```python
from build123d import *

# Parameters (mm, degrees)
BOSS_EXTRUDE1_DEPTH                             = 2
SKETCH2_R                                       = 4.4
CUT_EXTRUDE1_DEPTH                              = 34.661067402
CUT_EXTRUDE2_REACH                              = 35.661
SKETCH5_R                                       = 1.5
CSK_FOR_M2_FLAT_HEAD_MACHINE_SCREW1_D           = 2.4
CSK_FOR_M2_FLAT_HEAD_MACHINE_SCREW1_DEPTH       = 42.93
CSK_FOR_M2_FLAT_HEAD_MACHINE_SCREW1_CSINK_D     = 4.4
CSK_FOR_M2_FLAT_HEAD_MACHINE_SCREW1_CSINK_ANGLE = 90
CSK_FOR_M2_FLAT_HEAD_MACHINE_SCREW1_TIP         = 0.721032743
CSK_FOR_M2_FLAT_HEAD_MACHINE_SCREW2_D           = 2.4
CSK_FOR_M2_FLAT_HEAD_MACHINE_SCREW2_DEPTH       = 42.93
CSK_FOR_M2_FLAT_HEAD_MACHINE_SCREW2_CSINK_D     = 4.4
CSK_FOR_M2_FLAT_HEAD_MACHINE_SCREW2_CSINK_ANGLE = 90
CSK_FOR_M2_FLAT_HEAD_MACHINE_SCREW2_TIP         = 0.721032743


with BuildPart() as part:
    # Sketch1 → Boss-Extrude1 (new body)
    with BuildSketch(Plane(origin=(0, 0, 0), x_dir=(1, 0, 0), z_dir=(0, 1, 0))):
        Polygon((-11.293051345, 29.704532022), (12.706948655, 29.704532022), (15.706948655, 26.704532022), (15.706948655, 2.704532022), (12.706948655, -0.295467978), (-11.293051345, -0.295467978), (-14.293051345, 2.704532022), (-14.293051345, 26.704532022), align=None)
    extrude(amount=BOSS_EXTRUDE1_DEPTH)

    # Sketch2 → Cut-Extrude1 (cut, through all)
    with BuildSketch(Plane(origin=(0, 2, 0), x_dir=(1, 0, 0), z_dir=(0, 1, 0))):
        with Locations(Location((0, 14.704532022, 0), (0, 0, 270))):
            Circle(SKETCH2_R)
    extrude(amount=-CUT_EXTRUDE1_DEPTH, mode=Mode.SUBTRACT)

    # Sketch5 → Cut-Extrude2 (cut, up to next)
    with BuildSketch(Plane(origin=(0, 2, 0), x_dir=(1, 0, 0), z_dir=(0, 1, 0)), mode=Mode.PRIVATE) as cut_extrude2_sk1:
        with Locations(Location((-3.508440786, 20.204532022, 0), (0, 0, 270))):
            Circle(SKETCH5_R)
    cut_extrude2_tool1 = extrude(cut_extrude2_sk1.sketch, amount=-CUT_EXTRUDE2_REACH, mode=Mode.PRIVATE) & part.part
    # Sketch5 → Cut-Extrude2 (cut, up to next)
    with BuildSketch(Plane(origin=(0, 2, 0), x_dir=(1, 0, 0), z_dir=(0, 1, 0)), mode=Mode.PRIVATE) as cut_extrude2_sk2:
        with Locations(Location((3.491559214, 20.204532022, 0), (0, 0, 270))):
            Circle(SKETCH5_R)
    cut_extrude2_tool2 = extrude(cut_extrude2_sk2.sketch, amount=-CUT_EXTRUDE2_REACH, mode=Mode.PRIVATE) & part.part
    add(cut_extrude2_tool1.solids().sort_by_distance((-3.508441, 2, -20.204532))[0], mode=Mode.SUBTRACT)
    add(cut_extrude2_tool2.solids().sort_by_distance((3.491559, 2, -20.204532))[0], mode=Mode.SUBTRACT)

    # CSK for M2 Flat Head Machine Screw1
    with Locations(Plane(origin=(-3.508440786, 2, -20.204532022), x_dir=(0, 0, 1), z_dir=(0, 1, 0))):
        with Locations((0, 0), (0, 7)):
            CounterSinkHole(CSK_FOR_M2_FLAT_HEAD_MACHINE_SCREW1_D / 2, CSK_FOR_M2_FLAT_HEAD_MACHINE_SCREW1_CSINK_D / 2, depth=CSK_FOR_M2_FLAT_HEAD_MACHINE_SCREW1_DEPTH, counter_sink_angle=CSK_FOR_M2_FLAT_HEAD_MACHINE_SCREW1_CSINK_ANGLE)
            with Locations((0, 0, -(CSK_FOR_M2_FLAT_HEAD_MACHINE_SCREW1_DEPTH + CSK_FOR_M2_FLAT_HEAD_MACHINE_SCREW1_TIP / 2))):  # 118° drill point
                Cone(0, CSK_FOR_M2_FLAT_HEAD_MACHINE_SCREW1_D / 2, CSK_FOR_M2_FLAT_HEAD_MACHINE_SCREW1_TIP, mode=Mode.SUBTRACT)

    # CSK for M2 Flat Head Machine Screw2
    with Locations(Plane(origin=(0, 2, 0), x_dir=(1, 0, 0), z_dir=(0, 1, 0))):
        with Locations((-11.293051345, 26.704532022), (-11.293051345, 2.704532022), (12.706948655, 26.704532022), (12.706948655, 2.704532022)):
            CounterSinkHole(CSK_FOR_M2_FLAT_HEAD_MACHINE_SCREW2_D / 2, CSK_FOR_M2_FLAT_HEAD_MACHINE_SCREW2_CSINK_D / 2, depth=CSK_FOR_M2_FLAT_HEAD_MACHINE_SCREW2_DEPTH, counter_sink_angle=CSK_FOR_M2_FLAT_HEAD_MACHINE_SCREW2_CSINK_ANGLE)
            with Locations((0, 0, -(CSK_FOR_M2_FLAT_HEAD_MACHINE_SCREW2_DEPTH + CSK_FOR_M2_FLAT_HEAD_MACHINE_SCREW2_TIP / 2))):  # 118° drill point
                Cone(0, CSK_FOR_M2_FLAT_HEAD_MACHINE_SCREW2_D / 2, CSK_FOR_M2_FLAT_HEAD_MACHINE_SCREW2_TIP, mode=Mode.SUBTRACT)


solid = part.part
```
The listing builds one solid part. Answer for the finished solid, in the listing's coordinates (mm). Give positions to 0.01 mm unless a question says otherwise; leave off trailing zeros. Write each loop counter-clockwise with the first axis right and the second up, starting at its lowest first coordinate (ties: lowest second). Pieces come first, ordered by that corner, then holes. Notation, with made-up numbers: (68, -30.75) -> (101, -30.75) arc R20 ccw to (101, -15.75) -> close; hole circle Ø2 at (2, 65.5). An arc over 180 degrees is marked (long way). Use one line per item in the form item = value.
1) Section B-B on y = 0.35 is taken. Write down the section's boundary in (x, z).
Result:
outline = (-14.29, -26.7) -> (-11.29, -29.7) -> (12.71, -29.7) -> (15.71, -26.7) -> (15.71, -2.7) -> (12.71, 0.3) -> (-11.29, 0.3) -> (-14.29, -2.7) -> close; hole circle Ø2.4 at (-11.29, -26.7); hole circle Ø2.4 at (-11.29, -2.7); hole circle Ø3 at (-3.51, -20.2); hole circle Ø8.8 at (0, -14.7); hole circle Ø3 at (3.49, -20.2); hole circle Ø2.4 at (12.71, -26.7); hole circle Ø2.4 at (12.71, -2.7)
2) Each of these flat-tipped pins is pushed along its axis until it touches: P1, Ø3.5, axis at x = 3.49, z = -20.2, coming from the +Y side; P2, Ø3, axis at x = 12.71, z = -2.7, coming from the +Y side. Where does it stop, or does it pass through?
Result:
P1 = 1.55
P2 = 1.31
3) Section A-A on x = 0 is taken. Write down the section's boundary in (y, z).
Result:
outline = (0, -29.7) -> (2, -29.7) -> (2, -19.1) -> (0, -19.1) -> close; (0, -10.3) -> (2, -10.3) -> (2, 0.3) -> (0, 0.3) -> close
4) For a pull along X with two mould halves and no side action, classify faces 1 (the cylindrical face through (0.2, 1, -19.1)), 2 (the flat face through (-12.77, 0.99, -1.18)), 3 (the flat face through (14.186, 0.986, -28.226)) as +X half, -X half, draft (parallel to the pull), parting line (faces both ways), or undercut.
Result:
face_1 = undercut
face_2 = -X half
face_3 = +X half
5) Section C-C on x = 4 is taken. Count the separate pieces of the cut face and the enclosed holes in it, plus the area to 3 significant figures.
Result:
separate_pieces = 3
enclosed_holes = 0
area = 46.5 mm²
6) Straight lines are drawn through the part: probe 1 along Z at (x, y) = (4, 0.9); probe 2 along Z at (x, y) = (3.5, 1.8); probe 3 along X at (y, z) = (0.95, -26.75). For each, find the intervals that lie inside material, in ascending order.
Result:
probe_1 = -29.7 to -21.62, -18.79 to -16.54, -12.87 to 0.3
probe_2 = -29.7 to -22.2, -18.2 to -17.37, -12.04 to 0.3
probe_3 = -14.25 to -12.49, -10.09 to 11.51, 13.91 to 15.66
